Input: part model. Units: mm. Frame: model coordinates. A direction names the side the tool comes from. Coordinates: 2 decimals unless noted, no trailing zeros. Write each loop counter-clockwise with the first axis right and the second up, starting at its lowest first coordinate (ties: lowest second). Pieces come first, ordered by that corner, then holes.
1) Section query B-B (x = 19). Output: boundary loops of the cut face in (y, z), then the cut area to 3 significant figures.
2) Set-up query: faces 1 (the flat face through (23, 7, 23)), 2 (the flat face through (-17.168, 4, -28)), 3 (the flat face through (-17.168, 4, 36)), 4 (the cylindrical face through (34.996, 3.944, -0.519)). Return all of +Z, -Z, +X, -X, +Y, -Y with unobstructed straight access to the full face (end or side cutting, diameter ignored); none if empty.
3) Draft query along Z for faces 5 (the flat face through (-23, 7, 23)), 6 (the flat face through (0, 4, 40.5)), 7 (the flat face through (17.168, 4, 35)). Return one class per face: pulls with the +Z half, pulls with the -Z half, needs draft (parallel to the pull), parting line crosses it, or undercut.
4) Line query: L1, parallel to X at y = 7.5, z = 24; L2, parallel to X at y = 1.5, z = -1; L3, parallel to X at y = 7, z = 15. Output: solid intervals per line, ascending.
5) Section query C-C (y = 4.75). Output: boundary loops of the cut face in (x, z), then the cut area to 3 significant figures.
6) Section query A-A (z = -6.5). Output: boundary loops of the cut face in (x, y), then the cut area to 3 significant figures.
7) Pin query (flat end, axial travel): pin 1 Ø2.5 at (y, z) = (4.5, -28) entering from +X; pin 2 Ø2.5 at (y, z) = (3, 36.5) entering from +X; pin 3 Ø2.5 at (x, z) = (23.16, 23.16) entering from +Y; pin 4 Ø5 at (x, z) = (-23.16, -23.16) entering from -Y. Return the tip coordinate at first contact, or that it passes through.
8) Section query D-D (x = -5.5). Output: boundary loops of the cut face in (y, z), then the cut area to 3 significant figures.
Autodesk Inventor part; units mm, degrees
ref_plane "YZ Plane" through (0, 0, 0) normal (1, 0, 0) x (0, 1, 0)
ref_plane "XZ Plane" through (0, 0, 0) normal (0, 1, 0) x (-1, 0, 0)
ref_plane "XY Plane" through (0, 0, 0) normal (0, 0, 1) x (1, 0, 0)
sketch "Sketch1" plane through (0, 0, 0) normal (0, 1, 0) x (-1, 0, 0)
  circle A0 centre (0, 0) radius 35
  dimension "d0" = 70
extrude "Extrusion1" add sketch "Sketch1" along normal blind 8
sketch "Sketch2" plane through (0, 8, 0) normal (0, 1, 0) x (1, 0, 0)
  circle A0 centre (0, 0) radius 30.5
  dimension "d3" = 61
extrude "Extrusion2" cut sketch "Sketch2" against normal blind 8
sketch "Sketch3" plane through (0, 8, 0) normal (0, 1, 0) x (1, 0, 0)
  circle A0 centre (0, 0) radius 30.5
  line L0 (0, -30.5) -> (-17.1683, -30.5)
  circle A1 centre (0, 0) radius 35
  line L1 (-17.1683, -30.5) -> (17.1677, -30.5)
  line L2 (17.1677, -30.5) -> (17.1677, -40.5)
  line L3 (17.1677, -40.5) -> (-17.1683, -40.5)
  line L4 (-17.1683, -40.5) -> (-17.1683, -30.5)
  dimension "d6" = 34.336
  dimension "d7" = 10
extrude "Extrusion3" add sketch "Sketch3" against normal blind 8 contours L1 A1 L0 | A1 L2 L3 L4 picked at (9.255, -31.4525)
sketch "Sketch4" plane through (0, 8, 0) normal (0, 1, 0) x (1, 0, 0)
  line L0 (-17.1683, -40.5) -> (-17.1683, -30.5)
  line L1 (-17.1683, -30.5) -> (-17.1683, 30.5)
  arc A0 (17.1677, -30.5003) -> (-17.1683, -30.5) centre (0, 0) ccw
  line L2 (17.1677, -30.5003) -> (17.1677, 30.5)
  circle A1 centre (0, 0) radius 30.5
  line L3 (-17.1683, 25.2091) -> (17.1677, 25.2091)
  line L4 (17.1677, 25.2091) -> (17.1677, 37.2402)
  line L5 (17.1677, 37.2402) -> (-17.1683, 37.2402)
  line L6 (-17.1683, 37.2402) -> (-17.1683, 25.2091)
  point P0 (17.1677, 30.5)
extrude "Extrusion4" cut sketch "Sketch4" against normal blind 8 contours L1 A0 L2 A1 | A1 L3 | L6 L5 L4 A0
sketch "Sketch5" plane through (0, 8, 0) normal (0, 1, 0) x (1, 0, 0)
  point P0 (0, 0)
sketch "Sketch6" plane through (0, 8, 0) normal (0, 1, 0) x (1, 0, 0)
  line L0 (0, 0) -> (-23.1577, 23.1577)
  line L1 (0, 0) -> (32.75, 0) construction
  circle A0 centre (-23.1577, 23.1577) radius 1.5
  dimension "d12" = 32.75
  dimension "d13" = 135
  dimension "d14" = 3
extrude "Extrusion5" cut sketch "Sketch6" against normal blind 1
sketch "Sketch7" plane through (0, 8, 0) normal (0, 1, 0) x (1, 0, 0)
  line L0 (0, 0) -> (-23.1577, -23.1577)
  line L1 (0, 0) -> (32.75, 0) construction
  circle A0 centre (-23.1577, -23.1577) radius 1.5
  dimension "d17" = 32.75
  dimension "d18" = 135
  dimension "d19" = 3
extrude "Extrusion6" cut sketch "Sketch7" against normal blind 1
sketch "Sketch8" plane through (0, 8, 0) normal (0, 1, 0) x (1, 0, 0)
  line L0 (0, 0) -> (23.1577, -23.1577)
  line L1 (0, 0) -> (32.75, 0) construction
  circle A0 centre (23.1577, -23.1577) radius 1.5
  dimension "d22" = 32.75
  dimension "d23" = 45
  dimension "d24" = 3
extrude "Extrusion7" cut sketch "Sketch8" against normal blind 1
sketch "Sketch9" plane through (0, 8, 0) normal (0, 1, 0) x (1, 0, 0)
  line L0 (0, 0) -> (23.1577, 23.1577)
  line L1 (0, 0) -> (32.75, 0) construction
  circle A0 centre (23.1577, 23.1577) radius 1.5
  dimension "d27" = 32.75
  dimension "d28" = 45
  dimension "d29" = 3
extrude "Extrusion8" cut sketch "Sketch9" against normal blind 1
sketch "Sketch10" plane through (0, 8, 0) normal (0, 1, 0) x (1, 0, 0)
  point P0 (0, 0)
properties part number "expo5"
Answer:
1. outline: (0, -29.39) - (8, -29.39) - (8, -23.86) - (0, -23.86) - close; (0, 23.86) - (8, 23.86) - (8, 29.39) - (0, 29.39) - close
1. area: 88.6 mm2
2. face 1: +Y
2. face 2: -Z, +Y, -Y
2. face 3: +Z, -X, +Y, -Y
2. face 4: +X, +Y, -Y
3. face 5: undercut
3. face 6: pulls with the +Z half
3. face 7: needs draft
4. L1: x = -25.48 to -24.4, -21.92 to -18.82, 18.82 to 21.92, 24.4 to 25.48
4. L2: x = -34.99 to -30.48, 30.48 to 34.99
4. L3: x = -31.62 to -26.56, 26.56 to 31.62
5. outline: (-17.17, -30.5) - (-17.17, -25.21) arc R30.5 cw (long way) to (17.17, -25.21) - (17.17, -30.5) arc R35 ccw to (17.17, 30.5) - (17.17, 40.5) - (-17.17, 40.5) - (-17.17, 30.5) arc R35 ccw to start
5. area: 1,000 mm2
6. outline: (-34.39, 0) - (-29.8, 0) - (-29.8, 8) - (-34.39, 8) - close; (29.8, 0) - (34.39, 0) - (34.39, 8) - (29.8, 8) - close
6. area: 73.5 mm2
7. pin 1: stops at x = 22.57
7. pin 2: stops at x = 17.17
7. pin 3: stops at y = 7
7. pin 4: stops at y = 0
8. outline: (0, 30) - (8, 30) - (8, 40.5) - (0, 40.5) - close
8. area: 84.0 mm2
